```python
from build123d import *

# Parameters (mm, degrees)
SKETCH2_W               = 50.8
SKETCH2_H               = 36.83
BOSS_EXTRUDE1_DEPTH     = 8.89
SKETCH14_W              = 36.83
SKETCH14_H              = 8.89
BOSS_EXTRUDE6_DEPTH     = 0.254
SKETCH15_W              = 4.318
SKETCH15_H              = 10.16
BOSS_EXTRUDE7_DEPTH     = 20.32
CUT_EXTRUDE3_DEPTH      = 54.86357322
CUT_EXTRUDE3_DEPTH_BACK = 54.86357322
SKETCH16_R              = 2.54
FILLET1_R               = 3.81
SKETCH18_R              = 1.397
CUT_EXTRUDE5_DEPTH      = 2.286
SKETCH18_5_W            = 22.86
SKETCH18_5_H            = 4.572
CUT_EXTRUDE6_DEPTH      = 7.62
SKETCH18_6_W            = 22.86
SKETCH18_6_H            = 4.572
CUT_EXTRUDE7_DEPTH      = 7.62


with BuildPart() as part:
    # Sketch2 → Boss-Extrude1 (new body)
    with BuildSketch(Plane(origin=(0, 0, 0), x_dir=(1, 0, 0), z_dir=(0, 1, 0))):
        Rectangle(SKETCH2_W, SKETCH2_H)
    extrude(amount=-BOSS_EXTRUDE1_DEPTH)

    # Sketch14 → Boss-Extrude6 (add)
    with BuildSketch(Plane(origin=(25.4, 0, 0), x_dir=(0, 0, -1), z_dir=(1, 0, 0))):
        with Locations((0, -4.445)):
            Rectangle(SKETCH14_W, SKETCH14_H)
    extrude(amount=BOSS_EXTRUDE6_DEPTH)

    # Sketch15 → Boss-Extrude7 (add)
    with BuildSketch(Plane(origin=(25.654, 0, 0), x_dir=(0, 0, -1), z_dir=(1, 0, 0))):
        with Locations((-5.588, -5.08)):
            Rectangle(SKETCH15_W, SKETCH15_H)
        with Locations((5.588, -5.08)):
            Rectangle(SKETCH15_W, SKETCH15_H)
    extrude(amount=BOSS_EXTRUDE7_DEPTH)

    # Sketch16 → Cut-Extrude3 (cut, two sides: drawn at the far end of the back side and taken through both)
    with BuildSketch(Plane(origin=(0, 0, -7.747), x_dir=(-1, 0, 0), z_dir=(0, 0, -1)).offset(-CUT_EXTRUDE3_DEPTH_BACK)):
        with Locations((-40.894, -4.445)):
            Circle(SKETCH16_R)
    extrude(amount=CUT_EXTRUDE3_DEPTH + CUT_EXTRUDE3_DEPTH_BACK, mode=Mode.SUBTRACT)

    # Fillet1
    fillet1_edges = [part.edges().sort_by_distance(p)[0] for p in [
        (45.974, 0, 5.588),
        (45.974, -10.16, 5.588),
        (45.974, 0, -5.588),
        (45.974, -10.16, -5.588),
    ]]
    fillet(fillet1_edges, radius=FILLET1_R)

    # Sketch18 → Cut-Extrude5 (cut)
    with BuildSketch(Plane(origin=(0, 0, 0), x_dir=(1, 0, 0), z_dir=(0, 1, 0))):
        with Locations(Location((-19.05, -14.478, 0), (0, 0, 270))):
            Circle(SKETCH18_R)
        with Locations(Location((-19.05, 14.478, 0), (0, 0, 270))):
            Circle(SKETCH18_R)
    extrude(amount=-CUT_EXTRUDE5_DEPTH, mode=Mode.SUBTRACT)

    # Sketch18_5 → Cut-Extrude6 (cut)
    with BuildSketch(Plane(origin=(0, 0, 0), x_dir=(1, 0, 0), z_dir=(0, 1, 0))):
        with Locations((11.43, 15.24)):
            Rectangle(SKETCH18_5_W, SKETCH18_5_H)
    extrude(amount=-CUT_EXTRUDE6_DEPTH, mode=Mode.SUBTRACT)

    # Sketch18_6 → Cut-Extrude7 (cut)
    with BuildSketch(Plane(origin=(0, 0, 0), x_dir=(1, 0, 0), z_dir=(0, 1, 0))):
        with Locations((11.43, -15.24)):
            Rectangle(SKETCH18_6_W, SKETCH18_6_H)
    extrude(amount=-CUT_EXTRUDE7_DEPTH, mode=Mode.SUBTRACT)


solid = part.part
```
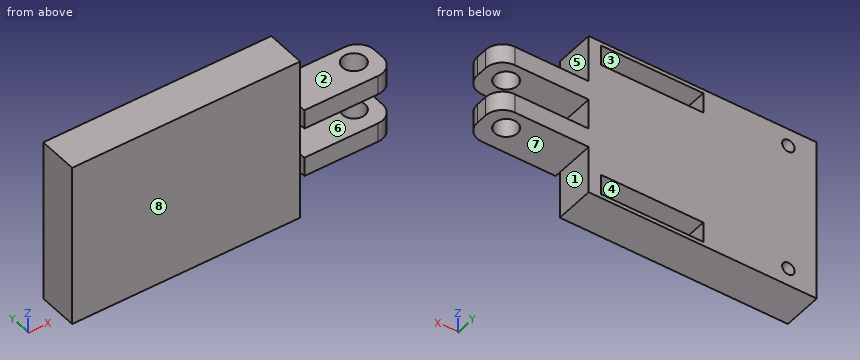
Verification items for the finished model (mm, model axes). Face numbers are marked on the shaded views. A direction names the side the tool comes from. Give positions to 0.01 mm unless a question says otherwise; leave off trailing zeros. Order: outer loops, then holes, each group sorted by start corner. A loop starts at its lowest first (then second) coordinate and runs counter-clockwise, first axis right, second up. Notation, with made-up numbers: (6, 6.5) -> (45, 6.5) arc R32 cw to (45, 41.5) -> close; hole circle Ø9 at (-4, 25). An arc over 180 degrees is marked (long way). One line per item, written item: value.
(1) Sectioned sample at D-D on x = 17.5. Record the cut outline in (y, z) (3 decimals), then the cut area to 3 significant figures.
Final values:
outline: (-8.89, -18.415) -> (0, -18.415) -> (0, -17.526) -> (-7.62, -17.526) -> (-7.62, -12.954) -> (0, -12.954) -> (0, 12.954) -> (-7.62, 12.954) -> (-7.62, 17.526) -> (0, 17.526) -> (0, 18.415) -> (-8.89, 18.415) -> close
area: 258 mm^2
(2) Sectioned sample at C-C on y = -3. Record the cut outline in (x, z) (3 decimals).
Final values:
outline: (-25.4, -18.415) -> (25.654, -18.415) -> (25.654, -7.747) -> (38.805, -7.747) -> (38.805, -3.429) -> (25.654, -3.429) -> (25.654, 3.429) -> (38.805, 3.429) -> (38.805, 7.747) -> (25.654, 7.747) -> (25.654, 18.415) -> (-25.4, 18.415) -> close; (42.983, -7.747) -> (45.887, -7.747) -> (45.887, -3.429) -> (42.983, -3.429) -> close; (42.983, 3.429) -> (45.887, 3.429) -> (45.887, 7.747) -> (42.983, 7.747) -> close; hole (0, -17.526) -> (22.86, -17.526) -> (22.86, -12.954) -> (0, -12.954) -> close; hole (0, 12.954) -> (22.86, 12.954) -> (22.86, 17.526) -> (0, 17.526) -> close
(3) Scan lines: line 1 along Z through (x, y) = (11, -5.5) (3 decimals); line 2 along X through (y, z) = (-4, 16.5); line 3 along Z through (x, y) = (37, -6.5). Record each from-to range of solid material in increasing order. Write a range as [from, to].
Final values:
line 1: [-18.415, -17.526], [-12.954, 12.954], [17.526, 18.415]
line 2: [-25.4, 0], [22.86, 25.65]
line 3: [-7.75, -3.43], [3.43, 7.75]
(4) Draft check along Z on the marked faces 1, 2 and 3. Enter one of: pulls with the +Z half, pulls with the -Z half, needs draft (parallel to the pull), parting line crosses it, or undercut.
Final values:
face 1: needs draft
face 2: pulls with the +Z half
face 3: undercut
(5) Sectioned sample at B-B on z = 5. Record the cut outline in (x, y) (3 decimals).
Final values:
outline: (-25.4, -8.89) -> (25.654, -8.89) -> (25.654, -10.16) -> (42.164, -10.16) arc R3.81 ccw to (45.974, -6.35) -> (45.974, -3.81) arc R3.81 ccw to (42.164, 0) -> (-25.4, 0) -> close; hole circle Ø5.08 at (40.894, -4.445)
(6) Tool access check on the marked faces 4, 5, 6, 7 and 8. Record the directions out of +Z, -Z, +X, -X, +Y, -Y that give a thin tool (end or side, any length) a straight path to the whole face; none if there is none.
Final values:
face 4: +Y
face 5: +Z, +X, +Y, -Y
face 6: +X, +Y, -Y
face 7: -Z, +X, +Y, -Y
face 8: +Z, -Z, -X, -Y
(7) Gauge pin test, flat ends, axial feed: pin 1 (2.5 mm diameter, centred on y = -3.5, z = -14, fed in from +X); pin 2 (2 mm diameter, centred on x = -17.5, z = -14.5, fed in from -Y); pin 3 (1 mm diameter, centred on y = -7, z = -3, fed in from +X). Record the tip position at first contact, or that the pin passes through.
Final values:
pin 1: x = 25.65
pin 2: y = -8.89
pin 3: x = 45.95
(8) Sectioned sample at A-A on x = 34. Record the cut outline in (y, z).
Final values:
outline: (-10.16, -7.75) -> (0, -7.75) -> (0, -3.43) -> (-10.16, -3.43) -> close; (-10.16, 3.43) -> (0, 3.43) -> (0, 7.75) -> (-10.16, 7.75) -> close
